```python
from build123d import *

# Parameters (mm, degrees)
F0_W     = 15
F0_H     = 30
F1_DEPTH = 25
F2_DEPTH = 50
F5_DEPTH = 23.6443121872
F7_DEPTH = 15


with BuildPart() as f1:
    # F0 (on Right) → F1 (new body)
    with BuildSketch(Plane.YZ):
        with Locations((22.5, 15)):
            Rectangle(F0_W, F0_H)
        Polygon((15, 30), (0, 0), (15, 0), align=None)
    extrude(amount=F1_DEPTH)

    # F0 (on Right) → F2 (join)
    with BuildSketch(Plane.YZ):
        with Locations((22.5, 15)):
            Rectangle(F0_W, F0_H)
    extrude(amount=F2_DEPTH)

    # F4 (on 3pt) → F5 (cut, through all)
    with BuildSketch(Plane(origin=(5.5900621118, -9.3167701863, 4.6583850932), x_dir=(-0.8811342211, -0.4229444261, 0.2114722131), z_dir=(-0.4728662437, 0.7881104062, -0.3940552031))):
        Polygon((-50.4008774448, 6.7082039325), (-22.0283555266, 33.5410196625), (-50.4008774448, 40.249223595), align=None)
    extrude(amount=-F5_DEPTH, mode=Mode.SUBTRACT)

    # F6 (on Front) → F7 (join)
    with BuildSketch(Plane.XZ):
        Polygon((25, 0), (50, 0), (50, 15), (25, 30), (0, 0), align=None)
    extrude(amount=-F7_DEPTH)


solid = f1.part
```
CAD build for the part. Positions are in the model's coordinates, mm. A direction names the side the tool comes from. Round coordinates to 2 decimals unless told otherwise and drop trailing zeros. Order: outer loops, then holes, each group sorted by start corner. A loop starts at its lowest first (then second) coordinate and runs counter-clockwise, first axis right, second up. Notation, with made-up numbers: (80, 71.5) -> (125, 71.5) arc R23 cw to (125, 104.5) -> close; hole circle Ø2 at (-7.5, 22). An arc over 180 degrees is marked (long way). One line per question, with ' | ' between items.
Q1. Probe probe 1 along Y at (x, z) = (39.5, 17); probe 2 along Y at (x, z) = (30.5, 26); probe 3 along Z at (x, y) = (15, 5.5). List the from-to ranges inside material, lowest first.
Completed:
probe 1: y = 0 to 15, 17.2 to 30 | probe 2: y = 0 to 15, 16.3 to 30 | probe 3: z = 0 to 18
Q2. Slice it at B-B (z = 28.5). Write the cut outline in (x, y), then the cut area to 3 significant figures.
Completed:
outline: (0, 14.25) -> (23.75, 14.25) -> (23.75, 0) -> (27.5, 0) -> (27.5, 15) -> (26.25, 15) -> (50, 29.25) -> (50, 30) -> (0, 30) -> close | area: 655 mm^2
Q3. Which spindle directions (+Z, -Z, +X, -X, +Y, -Y) get a long thin tool onto all of the face, cutting with end or side? Do faces 1 (the flat face through (25, 30, 15)), 2 (the flat face through (15.45, 5.73, 18.54)), 3 (the flat face through (37.67, 7.4, 22.4)). Say none if no direction does.
Completed:
face 1: +Z, -Z, +X, -X, +Y | face 2: +Z, -X, -Y | face 3: +Z, +X, -Y
Q4. Two-plate mould, pull along Y, no slides. Class faces 4 (the flat face through (43.231, 21.022, 20.168)), 5 (the flat face through (30, 0, 12)), 6 (the flat face through (41, 15, 15)), 7 (the flat face through (50, 26, 9)): released by +Y, released by -Y, zero draft, split by the parting line, or undercut.
Completed:
face 4: undercut | face 5: released by -Y | face 6: undercut | face 7: zero draft
Q5. Slice it at C-C (y = 25). Write the cut outline in (x, z).
Completed:
outline: (0, 0) -> (50, 0) -> (50, 20) -> (41.67, 30) -> (0, 30) -> close
Q6. Slice it at A-A (x = 27). Write the cut outline in (y, z), then the cut area to 3 significant figures.
Completed:
outline: (0, 0) -> (30, 0) -> (30, 30) -> (16.2, 30) -> (15, 27.6) -> (15, 28.8) -> (0, 28.8) -> close | area: 881 mm^2
Q7. Slice it at D-D (x = 40.5). Write the cut outline in (y, z), then the cut area to 3 significant figures.
Completed:
outline: (0, 0) -> (30, 0) -> (30, 30) -> (24.3, 30) -> (15, 11.4) -> (15, 20.7) -> (0, 20.7) -> close | area: 674 mm^2
Q8. Drop flat-ended pins along their axis: pin 1 (3 mm diameter, centred on y = 19, z = 26, fed in from +X); pin 2 (3 mm diameter, centred on x = 43, y = 13, fed in from +Z). Give the stop position or say it passes through.
Completed:
pin 1: stops at x = 37.8 | pin 2: stops at z = 20.1
